Model file for the job. Use its own axes, mm. A direction names the side the tool comes from. Coordinates: 2 decimals unless noted, no trailing zeros. Order: outer loops, then holes, each group sorted by start corner. A loop starts at its lowest first (then second) coordinate and runs counter-clockwise, first axis right, second up. Notation, with made-up numbers: (-21, 5.25) -> (23, 5.25) arc R14 ccw to (23, 31.25) -> close; hole circle Ø5 at (-18, 64.5). An arc over 180 degrees is marked (long way). Write item = value, one per line. Start each with the question number.
Q1. Wall check: line 1 (X direction, y = 2.75, z = -93); line 2 (X direction, y = 5.25, z = 13); line 3 (X direction, y = 18, z = -81). Give the ranges that are in metal, low to high. Write a range as from..to.
Q2. Flat gauge pins, fed straight in: pin 1 (2.5 mm diameter, centred on y = 15, z = 51, fed in from -X); pin 2 (2.5 mm diameter, centred on y = 12, z = 52.5, fed in from +X); pin 3 (2 mm diameter, centred on x = -10, y = 12, fed in from +Z). Where does each tip first touch, or does it go through?
Q3. Cut at A-A, the plane z = 36. List the corners of the cut face in (x, y), plus the area to 3 significant figures.
Q4. Cut at B-B, the plane y = 12. Give the number of separate pieces and of enclosed holes in the cut face, plus the area to 3 significant figures.
Q5. 3-axis set-ups, long thin cutter, end or side, ignore diameter. For faces 1 (the face through (-20.5, 13, 51)), 2 (the face through (11.7, 2, -95)), 3 (the face through (-15.71, 14.86, -69.75)), 4 (the face through (9, 12, 48.604)), 5 (the face through (-20.5, 12, -164)): which of +Z, -Z, +X, -X, +Y, -Y reach the whole face in a straight line?
Q6. Mould opens along Z. For faces 6 (the face through (-23.467, 12.325, -141.542)), 7 (the face through (0, 13, -159.469)), 8 (the face through (19.5, 12, -164)) say: +Z half, -Z half, draft (parallel to the pull), parting line (faces both ways), or undercut.
from build123d import *

# Parameters (mm, degrees)
SZKIC1_R                    = 1.35
SZKIC1_W                    = 24.4
SZKIC1_H                    = 45
DODANIE_WYCI_GNI_CIE1_DEPTH = 5
DODANIE_WYCI_GNI_CIE2_DEPTH = 25
WYTNIJ_WYCI_GNI_CIE5_DEPTH  = 26
SZKIC7_R                    = 1.35
WYTNIJ_WYCI_GNI_CIE6_DEPTH  = 46.852083325
SZKIC8_W                    = 8
SZKIC8_H                    = 5
SZKIC8_W_2                  = 9
DODANIE_WYCI_GNI_CIE3_DEPTH = 25


with BuildPart() as part:
    # Szkic1 → Dodanie-wyci_gni_cie1 (new body)
    with BuildSketch(Plane(origin=(0, 0, 0), x_dir=(1, 0, 0), z_dir=(0, 1, 0))):
        Polygon((10, 165.969204133), (14.5, 165.969204133), (14.5, 173.969204133), (19.5, 173.969204133), (19.5, 153.940017653), (25.352083325, 129.486424712), (25.352083325, -14.915125095), (19.5, -48.6036745), (-20.5, -48.6036745), (-26.352083325, -14.915125095), (-26.352083325, 129.486424712), (-20.5, 153.940017653), (-20.5, 173.969204133), (-15.5, 173.969204133), (-15.5, 165.969204133), (-11, 165.969204133), (-11, 173.969204133), (-5.495079248, 173.969204133), (-5.495079248, 165.969204133), (4.495079248, 165.969204133), (4.495079248, 173.969204133), (10, 173.969204133), align=None)
        with Locations((14.5, 109.8963255)):
            Circle(SZKIC1_R, mode=Mode.SUBTRACT)
        with Locations((14.5, 92.8963255)):
            Circle(SZKIC1_R, mode=Mode.SUBTRACT)
        with Locations((14.5, 75.8963255)):
            Circle(SZKIC1_R, mode=Mode.SUBTRACT)
        with Locations((8, 69.5963255)):
            Circle(SZKIC1_R, mode=Mode.SUBTRACT)
        with Locations((-9, 69.5963255)):
            Circle(SZKIC1_R, mode=Mode.SUBTRACT)
        with Locations((-15.5, 75.8963255)):
            Circle(SZKIC1_R, mode=Mode.SUBTRACT)
        with Locations((-15.5, 92.8963255)):
            Circle(SZKIC1_R, mode=Mode.SUBTRACT)
        with Locations((-15.5, 109.8963255)):
            Circle(SZKIC1_R, mode=Mode.SUBTRACT)
        with Locations((-0.5, 94.8963255)):
            Rectangle(SZKIC1_W, SZKIC1_H, mode=Mode.SUBTRACT)
    extrude(amount=DODANIE_WYCI_GNI_CIE1_DEPTH)

    # Szkic1_3 → Dodanie-wyci_gni_cie2 (add)
    with BuildSketch(Plane(origin=(0, 0, 0), x_dir=(1, 0, 0), z_dir=(0, 1, 0))):
        Polygon((14.5, 165.969204133), (10, 165.969204133), (10, 173.969204133), (4.495079248, 173.969204133), (4.495079248, 165.969204133), (-5.495079248, 165.969204133), (-5.495079248, 173.969204133), (-11, 173.969204133), (-11, 165.969204133), (-15.5, 165.969204133), (-15.5, 173.969204133), (-20.5, 173.969204133), (-20.5, 153.940017653), (-26.352083325, 129.486424712), (-26.352083325, -14.915125095), (-20.5, -48.6036745), (19.5, -48.6036745), (25.352083325, -14.915125095), (25.352083325, 129.486424712), (19.5, 153.940017653), (19.5, 173.969204133), (14.5, 173.969204133), align=None)
        Polygon((-13.2, 117.3963255), (-12.7, 117.3963255), (11.7, 117.3963255), (12.2, 117.3963255), (17.3, 112.070622628), (17.3, 72.7963255), (12.2, 66.7963255), (-13.2, 66.7963255), (-18.3, 72.7963255), (-18.3, 112.070622628), align=None, mode=Mode.SUBTRACT)
    extrude(amount=DODANIE_WYCI_GNI_CIE2_DEPTH)

    # Szkic6 → Wytnij-wyci_gni_cie5 (cut, through all)
    with BuildSketch(Plane(origin=(0, 25, 0), x_dir=(1, 0, 0), z_dir=(0, 1, 0))):
        Polygon((16.653559582, 59.7963255), (-17.653559582, 59.7963255), (-0.5, 39.615667168), align=None)
        Polygon((-21.352083325, 56.74466496), (-21.352083325, 16.848702414), (-3.763614868, 36.052349129), align=None)
        Polygon((2.763614868, 36.052349129), (20.352083325, 16.848702414), (20.352083325, 56.74466496), align=None)
        Polygon((17.161306881, -32.852341508), (20.352083325, -14.484074364), (20.352083325, 0.802588639), (2.931825406, -17.721341562), align=None)
        Polygon((15.206822662, -44.1036745), (16.091150305, -39.01288651), (-0.5, -21.370592599), (-17.091150305, -39.01288651), (-16.206822662, -44.1036745), align=None)
        Polygon((-0.5, -14.072090524), (20.352083325, 9.098992114), (-0.5, 32.212802226), (-21.352083325, 9.098992114), align=None)
        Polygon((-3.931825406, -17.721341562), (-21.352083325, 0.802588639), (-21.352083325, -14.484074364), (-18.161306881, -32.852341508), align=None)
        Polygon((11.240631704, 159.469204133), (-12.240631704, 159.469204133), (-0.5, 145.434029611), align=None)
        Polygon((-15.086387227, 155.078390111), (-15.5, 153.350062298), (-15.5, 128.192615569), (-3.790002176, 141.574284058), align=None)
        Polygon((14.5, 128.192615569), (14.5, 153.350062298), (14.086387227, 155.078390111), (2.790002176, 141.574284058), align=None)
        Polygon((-0.5, 137.741373143), (-12.177951744, 124.3963255), (11.177951744, 124.3963255), align=None)
    extrude(amount=-WYTNIJ_WYCI_GNI_CIE5_DEPTH, mode=Mode.SUBTRACT)

    # Szkic7 → Wytnij-wyci_gni_cie6 (cut, through all)
    with BuildSketch(Plane.ZY.offset(20.5)):
        with Locations((-171.169204133, 21)):
            Circle(SZKIC7_R)
        with Locations((-171.169204133, 4)):
            Circle(SZKIC7_R)
    extrude(amount=-WYTNIJ_WYCI_GNI_CIE6_DEPTH, mode=Mode.SUBTRACT)

    # Szkic8 → Dodanie-wyci_gni_cie3 (add)
    with BuildSketch(Plane(origin=(0, 25, 0), x_dir=(1, 0, 0), z_dir=(0, 1, 0))):
        Polygon((19.5, -52.255545309), (19.5, -48.6036745), (12.5, -48.6036745), (12.5, -53.6036745), (16.83, -53.6036745), align=None)
        with Locations((0.758846465, -51.1036745)):
            Rectangle(SZKIC8_W, SZKIC8_H)
        with Locations((-16, -51.1036745)):
            Rectangle(SZKIC8_W_2, SZKIC8_H)
    extrude(amount=-DODANIE_WYCI_GNI_CIE3_DEPTH)


solid = part.part
Here are the results:
q1.line_1 = -26.35..-16.85, -14.15..-12.7, 11.7..13.15, 15.85..25.35
q1.line_2 = -26.35..-21.35, -8.37..-1.46, 0.46..7.37, 20.35..25.35
q1.line_3 = -26.35..-18.3, 17.3..25.35
q2.pin_1 = -20.5
q2.pin_2 = 19.5
q2.pin_3 = 48.6
q3.outline = (-22.69, 0) -> (-14.26, 0) -> (-14.26, 25) -> (-22.69, 25) -> close; (13.26, 0) -> (21.69, 0) -> (21.69, 25) -> (13.26, 25) -> close
q3.area = 422 mm²
q4.separate_pieces = 1
q4.enclosed_holes = 12
q4.area = 5,470 mm²
q5.face_1 = +Z, -X, +Y, -Y
q5.face_2 = +Y, -Y
q5.face_3 = +Y
q5.face_4 = +Z, +Y, -Y
q5.face_5 = -Z, -X, +Y, -Y
q6.face_6 = -Z half
q6.face_7 = undercut
q6.face_8 = draft
